Geometry check sheet. Reference: the model listing, model coordinates, mm. A direction names the side the tool comes from. Give positions to 0.01 mm unless a question says otherwise; leave off trailing zeros. Write each loop counter-clockwise with the first axis right and the second up, starting at its lowest first coordinate (ties: lowest second). Pieces come first, ordered by that corner, then holes. Notation, with made-up numbers: M -5.5,76 L 37.5,76 A24 cw 37.5,104 Z; hole C -6,-15.75 d3. An arc over 180 degrees is marked long. Use one line per item in the form item = value. Start each with the question number.
```python
from build123d import *

# Parameters (mm, degrees)
SKETCH_1_R               = 17
SKETCH_1_R_2             = 14
EXTRUDE_1_DEPTH          = 10
SKETCH_2_W               = 38
SKETCH_2_H               = 38
EXTRUDE_2_DEPTH          = 22.5
SKETCH_3_W               = 32
SKETCH_3_H               = 32
CUT_EXTRUDE_1_DEPTH      = 19.5
SKETCH_4_R               = 14
CUT_EXTRUDE_2_DEPTH      = 36.046397818
SKETCH_5_W               = 38
SKETCH_5_H               = 38
SKETCH_5_W_2             = 12.1
SKETCH_5_H_2             = 11.16
EXTRUDE_3_DEPTH          = 3
SKETCH_6_R               = 1.5
EXTRUDE_4_DEPTH          = 3
SKETCH_7_R               = 1.5
EXTRUDE_5_DEPTH          = 5
CUT_EXTRUDE_3_DEPTH      = 2
CUT_EXTRUDE_5_DEPTH      = 43.16930163
CUT_EXTRUDE_5_DEPTH_BACK = 43.16930163
SKETCH_9_W               = 31.856814276
SKETCH_9_H               = 55.588041179


with BuildPart() as part:
    # 草图1 → 凸台-拉伸1 (new body)
    with BuildSketch(Plane.XY):
        Circle(SKETCH_1_R)
        Circle(SKETCH_1_R_2, mode=Mode.SUBTRACT)
    extrude(amount=EXTRUDE_1_DEPTH)

    # 草图2 → 凸台-拉伸2 (add)
    with BuildSketch(Plane(origin=(0, 0, 0), x_dir=(-1, 0, 0), z_dir=(0, 0, -1))):
        Rectangle(SKETCH_2_W, SKETCH_2_H)
    extrude(amount=EXTRUDE_2_DEPTH)

    # 草图3 → 切除-拉伸1 (cut)
    with BuildSketch(Plane(origin=(0, 0, -22.5), x_dir=(-1, 0, 0), z_dir=(0, 0, -1))):
        Rectangle(SKETCH_3_W, SKETCH_3_H)
    extrude(amount=-CUT_EXTRUDE_1_DEPTH, mode=Mode.SUBTRACT)

    # 草图4 → 切除-拉伸2 (cut, through all)
    with BuildSketch(Plane.XY):
        Circle(SKETCH_4_R)
    extrude(amount=-CUT_EXTRUDE_2_DEPTH, mode=Mode.SUBTRACT)

    # 草图5 → 凸台-拉伸3 (add)
    with BuildSketch(Plane(origin=(0, 0, -22.5), x_dir=(-1, 0, 0), z_dir=(0, 0, -1))):
        Rectangle(SKETCH_5_W, SKETCH_5_H)
        with Locations((1.55, -10.42)):
            Rectangle(SKETCH_5_W_2, SKETCH_5_H_2, mode=Mode.SUBTRACT)
    extrude(amount=-EXTRUDE_3_DEPTH)

    # 草图6 → 凸台-拉伸4 (add, symmetric)
    with BuildSketch(Plane(origin=(0, 0, 0), x_dir=(0, 0, -1), z_dir=(1, 0, 0))):
        with BuildLine():
            Line((22.5, 4.5), (25.5, 4.5))
            ThreePointArc((25.5, 4.5), (30, 0), (25.5, -4.5))
            Line((25.5, -4.5), (22.5, -4.5))
            Line((22.5, -4.5), (22.5, 4.5))
        make_face()
        with Locations((25.5, 0)):
            Circle(SKETCH_6_R, mode=Mode.SUBTRACT)
    extrude(amount=EXTRUDE_4_DEPTH, both=True)

    # 草图7 → 凸台-拉伸5 (add)
    # profile 1 of 2: a face of its own
    with BuildSketch(Plane(origin=(19, 0, 0), x_dir=(0, 0, -1), z_dir=(1, 0, 0))):
        with BuildLine():
            Line((22.5, 15), (26.5, 15))
            ThreePointArc((26.5, 15), (31.5, 10), (26.5, 5))
            Line((26.5, 5), (22.5, 5))
            Line((22.5, 5), (22.5, 15))
        make_face()
        with Locations((26.5, 10)):
            Circle(SKETCH_7_R, mode=Mode.SUBTRACT)
    # profile 2 of 2: a face of its own
    with BuildSketch(Plane(origin=(19, 0, 0), x_dir=(0, 0, -1), z_dir=(1, 0, 0))):
        with BuildLine():
            Line((22.5, -5), (22.5, -15))
            Line((22.5, -15), (26.5, -15))
            ThreePointArc((26.5, -15), (31.5, -10), (26.5, -5))
            Line((26.5, -5), (22.5, -5))
        make_face()
        with Locations(Location((26.5, -10, 0), (0, 0, 180))):
            Circle(SKETCH_7_R, mode=Mode.SUBTRACT)
    extrude_5 = extrude(amount=-EXTRUDE_5_DEPTH)

    # 草图8 → 切除-拉伸3 (cut)
    with BuildSketch(Plane.ZY.offset(-14)):
        Polygon((-26.5, 6.824573519), (-23.75, 8.41228676), (-23.75, 11.58771324), (-26.5, 13.175426481), (-29.25, 11.58771324), (-29.25, 8.41228676), align=None)
        Polygon((-29.25, -8.41228676), (-26.5, -6.824573519), (-23.75, -8.41228676), (-23.75, -11.58771324), (-26.5, -13.175426481), (-29.25, -11.58771324), align=None)
    cut_extrude_3 = extrude(amount=-CUT_EXTRUDE_3_DEPTH, mode=Mode.SUBTRACT)

    # 镜向1: 凸台-拉伸5, 切除-拉伸3 across plane
    add(extrude_5.mirror(Plane(origin=(0, 0, 0), x_dir=(0, 0, 1), z_dir=(1, 0, 0))))
    add(cut_extrude_3.mirror(Plane(origin=(0, 0, 0), x_dir=(0, 0, 1), z_dir=(1, 0, 0))), mode=Mode.SUBTRACT)

    # 草图9 → 切除-拉伸5 (cut, two sides: drawn at the far end of the back side and taken through both)
    with BuildSketch(Plane(origin=(0, 0, -22.5), x_dir=(-1, 0, 0), z_dir=(0, 0, -1)).offset(-CUT_EXTRUDE_5_DEPTH_BACK)):
        with Locations((15.928407138, -0.196580563)):
            Rectangle(SKETCH_9_W, SKETCH_9_H)
    extrude(amount=CUT_EXTRUDE_5_DEPTH + CUT_EXTRUDE_5_DEPTH_BACK, mode=Mode.SUBTRACT)


solid = part.part
```
(1) Thickness scan on probe 1 along Y at (x, z) = (18.2, -26.5); probe 2 along Y at (x, z) = (12, -5); probe 3 along Z at (x, y) = (2, 0). Record the ranges inside material, lowest first. Write a range as [from, to].
(2) Depth check by flat-ended pin: pin 1 (2 mm diameter, centred on y = -13.5, z = -24.5, fed in from -X); pin 2 (4.5 mm diameter, centred on x = 16.5, z = -24, fed in from -Y); pin 3 (8 mm diameter, centred on y = -3.5, z = -13.5, fed in from -X); pin 4 (1.6 mm diameter, centred on x = 15.5, y = 9.5, fed in from +Z). Enter the tip coordinate at first touch or a pass-through.
(3) Tool access check on faces 4 (the cylindrical face through (17, 0, 5)), 5 (the flat face through (14.986, 12.37, -25.106)), 6 (the flat face through (14, 12, -29)), 7 (the flat face through (4.5, -10, -21)). Record the directions out of +Z, -Z, +X, -X, +Y, -Y that give a thin tool (end or side, any length) a straight path to the whole face; none if there is none.
(4) Sectioned sample at C-C, the plane z = -21. Record the boundary of the cut face in (x, y), plus the area to 3 significant figures.
(5) Sectioned sample at A-A, the plane y = 0. Record the boundary of the cut face in (x, z), plus the area to 3 significant figures.
(6) Sectioned sample at D-D, the plane x = 10.5. Record the boundary of the cut face in (y, z).
(7) Sectioned sample at B-B, the plane z = -26. State how many separate pieces and enclosed holes the cut face has, plus the area to 3 significant figures.
(8) Draft check along Y on faces 1 (the flat face through (14.986, 7.63, -27.894)), 2 (the flat face through (19, 0, -12)), 3 (the cylindrical face through (2, 0, -30)). Enter one of: released by +Y, released by -Y, zero draft, split by the parting line, or undercut.
Numbers:
q1.probe_1 = [-15, -11.5], [-8.5, -5], [5, 8.5], [11.5, 15]
q1.probe_2 = [-19, -16], [16, 19]
q1.probe_3 = [-30, -27], [-24, -19.5]
q2.pin_1 = 14
q2.pin_2 = -19
q2.pin_3 = 16
q2.pin_4 = 0
q3.face_4 = +Z, +X
q3.face_5 = -X
q3.face_6 = -Z, -X, +Y, -Y
q3.face_7 = -Z, -X
q4.outline = M 0,-19 L 19,-19 L 19,19 L 0,19 L 0,-4.84 L 4.5,-4.84 L 4.5,-16 L 0,-16 Z
q4.area = 672 mm2
q5.outline = M 0,-30 L 3,-30 L 3,-27 L 0,-27 Z; M 0,-24 L 3,-24 L 3,-22.5 L 19,-22.5 L 19,0 L 17,0 L 17,10 L 14,10 L 14,-3 L 16,-3 L 16,-19.5 L 0,-19.5 Z
q5.area = 165 mm2
q6.outline = M -19,-22.5 L 19,-22.5 L 19,0 L 13.37,0 L 13.37,10 L 9.26,10 L 9.26,-3 L 16,-3 L 16,-19.5 L -16,-19.5 L -16,-3 L -9.26,-3 L -9.26,10 L -13.37,10 L -13.37,0 L -19,0 Z
q7.separate_pieces = 6
q7.enclosed_holes = 0
q7.area = 78.3 mm2
q8.face_1 = undercut
q8.face_2 = zero draft
q8.face_3 = split by the parting line
